The figure shows three views and two pictorial views of one solid part (mm, origin at its lowest corner). Answer the questions. A direction names the side the tool comes from. Coordinates: 2 decimals unless noted, no trailing zeros. Loops run counter-clockwise (first coordinate to the right, second up) from the corner with the lowest first, then second, coordinate; pieces in that order, holes last. Notation, with made-up numbers: M 42,65 L 62,65 A17 cw 62,69 Z; hole C -37.75,8.25 d7. An arc over 180 degrees is marked long. One line per item, written item: value. Start each with the question number.
1. The part is cut by section D-D (y = 25). Write down the section's boundary in (x, z) (1 decimal).
2. Flat-ended cylindrical pins translate along their axes: pin 1 (3 mm diameter, centred on x = 32.5, z = 21.5, fed in from -Y); pin 2 (3 mm diameter, centred on x = 35.3, y = 19.8, fed in from -Z); pin 3 (4 mm diameter, centred on y = 6, z = 69.5, fed in from +X) (1 decimal). Find the tip coordinate at first contact, or state that the pin passes through.
3. The part is cut by section C-C (z = 12). Write down the section's boundary in (x, y), then the cut area to 3 significant figures.
4. The part is cut by section B-B (x = 19.8). Write down the section's boundary in (y, z).
5. The part is cut by section A-A (y = 19.8). Write down the section's boundary in (x, z), then the cut area to 3 significant figures.
6. Consider probe 1 along Y at (x, z) = (12.05, 27); probe 2 along Z at (x, y) = (9.5, 17); probe 3 along X at (y, z) = (19, 27) (1 decimal). Determine where each line is inside the solid, lowest interval first.
7. For the marked faces 1, 2 and 3, determine the directions among +Z, -Z, +X, -X, +Y, -Y from which every point of the face is accessible in a straight line to the end or side of a thin tool.
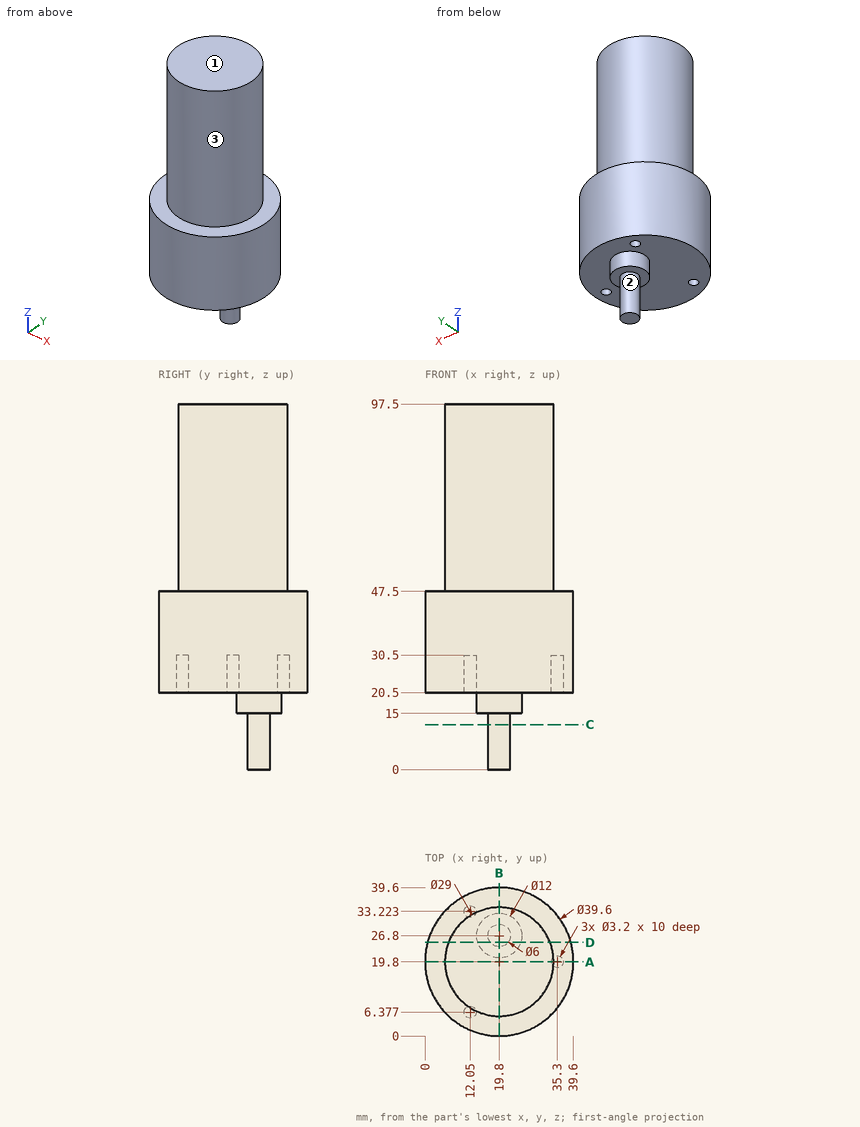
Answer block:
1. outline: M 0.7,20.5 L 14.1,20.5 L 14.1,15 L 17.4,15 L 17.4,0 L 22.2,0 L 22.2,15 L 25.5,15 L 25.5,20.5 L 38.9,20.5 L 38.9,47.5 L 33.3,47.5 L 33.3,97.5 L 6.3,97.5 L 6.3,47.5 L 0.7,47.5 Z
2. pin 1: stops at y = 3.47
2. pin 2: stops at z = 30.5
2. pin 3: stops at x = 28.2
3. outline: C 19.8,26.8 d6
3. area: 28.3 mm2
4. outline: M 0,20.5 L 20.8,20.5 L 20.8,15 L 23.8,15 L 23.8,0 L 29.8,0 L 29.8,15 L 32.8,15 L 32.8,20.5 L 39.6,20.5 L 39.6,47.5 L 34.3,47.5 L 34.3,97.5 L 5.3,97.5 L 5.3,47.5 L 0,47.5 Z
5. outline: M 0,20.5 L 33.7,20.5 L 33.7,30.5 L 36.9,30.5 L 36.9,20.5 L 39.6,20.5 L 39.6,47.5 L 34.3,47.5 L 34.3,97.5 L 5.3,97.5 L 5.3,47.5 L 0,47.5 Z
5. area: 2,490 mm2
6. probe 1: y = 1.58 to 4.78, 7.98 to 31.62, 34.82 to 38.02
6. probe 2: z = 20.5 to 97.5
6. probe 3: x = 0 to 33.9, 36.7 to 39.6
7. face 1: +Z, +X, -X, +Y, -Y
7. face 2: -Z
7. face 3: +Z
